from build123d import *

# Parameters (mm, degrees)
F1_DEPTH = 4.75
F2_R     = 1.45
F3_DEPTH = 18


with BuildPart() as f1:
    # F0 (on Front) → F1 (new body)
    with BuildSketch(Plane.XZ):
        Polygon((0, 64.8), (0, 0), (80.2, 0), (80.2, 33), (97.5, 33), (97.5, 64.8), align=None)
    extrude(amount=F1_DEPTH)

    # F2 (on face) → F3 (cut)
    with BuildSketch(Plane.XY.offset(64.8)):
        with Locations((89.5, -2.375)):
            Circle(F2_R)
        with BuildLine():
            ThreePointArc((6.55, -2.375), (8, -3.825), (9.45, -2.375))
            ThreePointArc((9.45, -2.375), (8, -0.925), (6.55, -2.375))
        make_face()
    extrude(amount=-F3_DEPTH, mode=Mode.SUBTRACT)


solid = f1.part
The model under review builds one solid part; all positions refer to its coordinate system, in mm. A direction names the side the tool comes from. Round coordinates to 2 decimals unless told otherwise and drop trailing zeros. Write each loop counter-clockwise with the first axis right and the second up, starting at its lowest first coordinate (ties: lowest second). Pieces come first, ordered by that corner, then holes. Notation, with made-up numbers: (58, 33) -> (98, 33) arc R8 cw to (98, 41) -> close; hole circle Ø10 at (-32.5, -5.5). An arc over 180 degrees is marked (long way). Answer as a JSON object with one key per item and string values.
1. The part is to be moulded in two halves that separate along X. For faces 4 (the face through (89, -2, 33)), 5 (the face through (0, -2, 33)), 6 (the face through (89, -2, 46.8)), say which applies: pulls with the +X half, pulls with the -X half, needs draft (parallel to the pull), parting line crosses it, or undercut.
Results found:
{"face 4": "needs draft", "face 5": "pulls with the -X half", "face 6": "undercut"}
2. Machinability: for faces 1 (the face through (8, -2, 46.8)), 2 (the face through (48, -4.75, 33)), 3 (the face through (80.2, -2, 16)), which of the approach directions +Z, -Z, +X, -X, +Y, -Y give a long, thin tool a straight path to every point of the face, cutting with its end or side? Answer none if there is none.
Results found:
{"face 1": "+Z", "face 2": "+Z, -Z, +X, -X, -Y", "face 3": "-Z, +X, +Y, -Y"}
3. We need section A-A on x = 8. State the section outline as (y, z) points (3 decimals).
Results found:
{"outline": "(-4.75, 0) -> (0, 0) -> (0, 64.8) -> (-0.925, 64.8) -> (-0.925, 46.8) -> (-3.825, 46.8) -> (-3.825, 64.8) -> (-4.75, 64.8) -> close"}
4. We need section C-C on x = 89.5. State the section outline as (y, z) points (3 decimals), and give its area (4 significant figures).
Results found:
{"outline": "(-4.75, 33) -> (0, 33) -> (0, 64.8) -> (-0.925, 64.8) -> (-0.925, 46.8) -> (-3.825, 46.8) -> (-3.825, 64.8) -> (-4.75, 64.8) -> close", "area": "98.85 mm^2"}
5. We need section B-B on z = 26. State the section outline as (x, y) points, and give its area (3 significant figures).
Results found:
{"outline": "(0, -4.75) -> (80.2, -4.75) -> (80.2, 0) -> (0, 0) -> close", "area": "381 mm^2"}
6. To check wall thickness, follow line 1 along Y through (x, z) = (89.5, 51.25) (3 decimals); line 2 along X through (y, z) = (-4.05, 26); line 3 along Z through (x, y) = (89.5, -1.8). State the ranges of each line that lie inside material, in increasing order.
Results found:
{"line 1": "y = -4.75 to -3.825, -0.925 to 0", "line 2": "x = 0 to 80.2", "line 3": "z = 33 to 46.8"}
7. Clearance check with flat-ended pins moving along their axes: pin 1 (1.7 mm diameter, centred on x = 89.5, y = -2.375, fed in from -Z); pin 2 (1.5 mm diameter, centred on x = 89, y = -2, fed in from +Z). State where each tip first meets the part, or that it passes through.
Results found:
{"pin 1": "stops at z = 33", "pin 2": "stops at z = 46.8"}
